Source: CAD feature listing. Evaluate the final solid. Frame: model axes, mm. Face numbers are marked on the shaded views. A direction names the side the tool comes from. Round coordinates to 2 decimals unless told otherwise and drop trailing zeros. Order: outer loops, then holes, each group sorted by start corner. A loop starts at its lowest first (then second) coordinate and runs counter-clockwise, first axis right, second up. Notation, with made-up numbers: (39, 2) - (73, 2) arc R26 ccw to (73, 22) - close; hole circle Ø10 at (-37, 27). An arc over 180 degrees is marked (long way). Use one line per item in the form item = value. Start each with the question number.
Q1. Pin query (flat end, axial travel): pin 1 Ø2 at (y, z) = (1.5, 1.5) entering from +X; pin 2 Ø3.5 at (x, z) = (0, -6) entering from +Y; pin 3 Ø3 at (y, z) = (2.5, 3) entering from +X. Return the tip coordinate at first contact, or that it passes through.
Q2. Ray query, line 1 (Z direction, x = 0, y = 7.55); line 2 (Z direction, x = 0, y = 4); line 3 (X direction, y = 4, z = 0). Return the intervals inside material, ascending. Write a range as [from, to].
Q3. Cut plane C-C, the plane y = 6. Return the cut outline in (x, z).
Q4. Cut plane D-D, the plane z = -6. Return the cut outline in (x, y).
Q5. Cut plane A-A, the plane x = 0. Return the cut outline in (y, z), and give its area (3 significant figures).
Q6. Set-up query: the marked faces 1 and 2. Return all of +Z, -Z, +X, -X, +Y, -Y with unobstructed straight access to the full face (end or side cutting, diameter ignored); none if empty.
Q7. Cut plane B-B, the plane z = 0. Return the cut outline in (x, y).
Q8. Draft query along X for the marked faces 3, 4 and 5. Return one class per face: released by +X, released by -X, zero draft, split by the parting line, or undercut.
Autodesk Inventor part; units mm, degrees
ref_plane "YZ Plane" through (0, 0, 0) normal (1, 0, 0) x (0, 1, 0)
ref_plane "XZ Plane" through (0, 0, 0) normal (0, 1, 0) x (-1, 0, 0)
ref_plane "XY Plane" through (0, 0, 0) normal (0, 0, 1) x (1, 0, 0)
sketch "Szkic1" plane through (0, 0, 0) normal (0, 1, 0) x (-1, 0, 0)
  circle A0 centre (0, 0) radius 15
  dimension "d0" = 30
extrude "Wyciągnięcie proste1" add sketch "Szkic1" along normal blind 2
sketch "Szkic2" plane through (0, 2, 0) normal (0, 1, 0) x (1, 0, 0)
  circle A0 centre (0, 0) radius 12.5
  dimension "d3" = 25
extrude "Wyciągnięcie proste2" add sketch "Szkic2" along normal blind 6
sketch "Szkic3" plane through (0, 8, 0) normal (0, 1, 0) x (1, 0, 0)
  circle A0 centre (0, -6) radius 1.45
  circle A1 centre (0, 6) radius 1.45
  point P0 (0, 0)
  dimension "d6" = 2.9
  dimension "d7" = 2.9
extrude "Wyciągnięcie proste3" cut sketch "Szkic3" against normal blind 8
sketch "Szkic4" plane through (0, 0, 0) normal (0, -1, 0) x (1, 0, 0)
  arc A0 (2.12, 1.59) -> (2.12, -1.59) centre (0, 0) ccw
  line L0 (2.12, 1.59) -> (2.12, -1.59)
  dimension "d10" = 5.3
  dimension "d11" = 2.12
extrude "Wyciągnięcie proste4" cut sketch "Szkic4" against normal blind 7
sketch "Szkic5" plane through (0, 8, 0) normal (0, 1, 0) x (1, 0, 0)
  circle A0 centre (0, -6) radius 1.45
  circle A1 centre (0, -6) radius 3
  circle A2 centre (0, 6) radius 1.45
  circle A3 centre (0, 6) radius 3
  point P0 (0, 0)
  dimension "d14" = 6
  dimension "d15" = 6
extrude "Wyciągnięcie proste5" cut sketch "Szkic5" against normal blind 1
properties part number "_Drukowanie 3D"
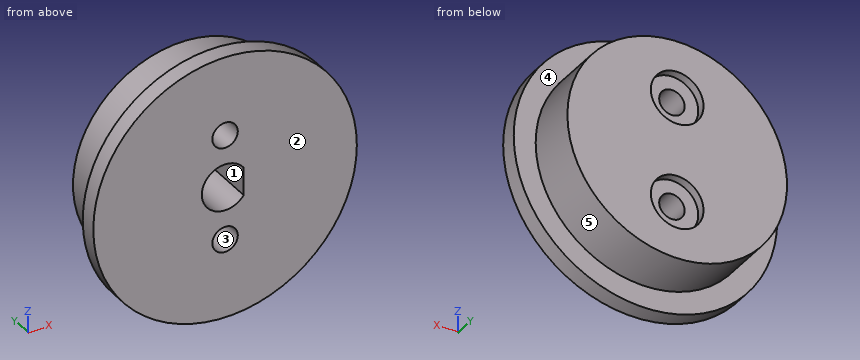
Completed:
q1.pin_1 = 14.99
q1.pin_2 = 7
q1.pin_3 = 14.92
q2.line_1 = [-12.5, -9], [-3, 3], [9, 12.5]
q2.line_2 = [-12.5, -7.45], [-4.55, -2.65], [2.65, 4.55], [7.45, 12.5]
q2.line_3 = [-12.5, -2.65], [2.12, 12.5]
q3.outline = circle Ø25 at (0, 0); hole circle Ø2.9 at (0, -6); hole circle Ø2.9 at (0, 6); hole (2.12, -1.59) - (2.12, 1.59) arc R2.65 ccw (long way) to start
q4.outline = (-13.75, 0) - (-1.45, 0) - (-1.45, 7) - (-3, 7) - (-3, 8) - (-10.97, 8) - (-10.97, 2) - (-13.75, 2) - close; (1.45, 0) - (13.75, 0) - (13.75, 2) - (10.97, 2) - (10.97, 8) - (3, 8) - (3, 7) - (1.45, 7) - close
q5.outline = (0, -15) - (2, -15) - (2, -12.5) - (8, -12.5) - (8, -9) - (7, -9) - (7, -7.45) - (0, -7.45) - close; (0, -4.55) - (7, -4.55) - (7, -3) - (8, -3) - (8, 3) - (7, 3) - (7, 4.55) - (0, 4.55) - (0, 2.65) - (7, 2.65) - (7, -2.65) - (0, -2.65) - close; (0, 7.45) - (7, 7.45) - (7, 9) - (8, 9) - (8, 12.5) - (2, 12.5) - (2, 15) - (0, 15) - close
q5.area = 120 mm2
q6.face_1 = -Y
q6.face_2 = +Z, -Z, +X, -X, -Y
q7.outline = (-15, 0) - (-2.65, 0) - (-2.65, 7) - (2.12, 7) - (2.12, 0) - (15, 0) - (15, 2) - (12.5, 2) - (12.5, 8) - (-12.5, 8) - (-12.5, 2) - (-15, 2) - close
q8.face_3 = undercut
q8.face_4 = zero draft
q8.face_5 = split by the parting line
